Autodesk Inventor part; units mm, degrees
ref_plane "YZ Plane" through (0, 0, 0) normal (1, 0, 0) x (0, 1, 0)
ref_plane "XZ Plane" through (0, 0, 0) normal (0, 1, 0) x (-1, 0, 0)
ref_plane "XY Plane" through (0, 0, 0) normal (0, 0, 1) x (1, 0, 0)
sketch "Sketch1" plane through (0, 0, 0) normal (0, 1, 0) x (-1, 0, 0)
  circle A0 centre (0, 0) radius 1.651
  circle A1 centre (0, -101.1428) radius 1.651
  line L0 (0, 0) -> (0, -101.1428) construction
  line L1 (3.175, 3.175) -> (-6.35, 3.175)
  line L2 (-6.35, 3.175) -> (-6.35, -104.3178)
  line L3 (-6.35, -104.3178) -> (3.175, -104.3178)
  line L4 (3.175, -104.3178) -> (3.175, 3.175)
  dimension "d0" = 3.302
  dimension "d1" = 101.1428
  dimension "d3" = 3.175
  dimension "d4" = 3.175
  dimension "d5" = 3.175
  dimension "d6" = 6.35
extrude "Extrusion1" add sketch "Sketch1" along normal blind 3.175
sketch "Sketch2" plane through (0, 0, 0) normal (0, -1, 0) x (1, 0, 0)
  line L0 (6.35, 3.175) -> (6.35, -104.3178)
  line L1 (6.35, -31.5214) -> (3.175, -31.5214)
  line L2 (3.175, -31.5214) -> (3.175, -69.6214)
  line L3 (3.175, -69.6214) -> (6.35, -69.6214)
  line L4 (6.35, -69.6214) -> (6.35, -31.5214)
  line L5 (-3.175, -104.3178) -> (-3.175, 3.175) construction
  line L6 (-3.175, -50.5714) -> (6.35, -50.5714) construction
  point P0 (0, 0)
  dimension "d9" = 38.1
  dimension "d10" = 3.175
extrude "Extrusion2" add sketch "Sketch2" along normal blind 41.275
sketch "Sketch3" plane through (6.35, 0, -104.3178) normal (1, 0, 0) x (0, 0, -1)
  circle A0 centre (-70.5866, -39.0652) radius 1.27
  circle A1 centre (-70.5866, -11.5697) radius 1.27
  circle A2 centre (-36.9062, -11.5697) radius 1.27
  circle A3 centre (-36.9062, -39.0652) radius 1.27
  line L0 (-70.5866, -11.5697) -> (-70.5866, -39.0652) construction
  line L1 (-70.5866, -39.0652) -> (-36.9062, -39.0652) construction
  line L2 (-36.9062, -39.0652) -> (-36.9062, -11.5697) construction
  line L3 (-36.9062, -11.5697) -> (-70.5866, -11.5697) construction
  line L4 (-34.6964, -41.275) -> (-72.7964, -41.275) construction
  line L5 (-53.7464, -41.275) -> (-53.7464, 0) construction
  line L6 (-34.6964, 0) -> (-72.7964, 0) construction
  line L7 (-68.3768, -41.275) -> (-39.116, -41.275)
  line L8 (-39.116, -41.275) -> (-39.116, -3.175)
  line L9 (-39.116, -3.175) -> (-68.3768, -3.175)
  line L10 (-68.3768, -3.175) -> (-68.3768, -41.275)
  line L11 (-72.7964, 0) -> (-72.7964, -41.275)
  point P0 (-104.3178, 0)
  dimension "d13" = 2.54
  dimension "d14" = 27.4955
  dimension "d15" = 33.6804
  dimension "d17" = 2.2098
  dimension "d18" = 2.2098
  dimension "d19" = 2.2098
  dimension "d20" = 2.2098
  dimension "d21" = 3.175
extrude "Extrusion3" cut sketch "Sketch3" against normal up to surface (3.175 mm away)
chamfer "Chamfer1" distance 6.35 angle 45 1 edges at (3.175, 0, -50.5714)
chamfer "Chamfer2" distance 3.175 distance2 34.6964 1 edges at (6.35, 1.5875, 3.175) measured on face at (0, 1.0583, 3.175)
chamfer "Chamfer3" distance 34.6964 distance2 3.175 1 edges at (6.35, 1.5875, -104.3178) measured on face at (6.35, 2.1167, -68.4869)
properties part number "grumpy camera mount"
Can you work these out from the model? Positions are in its coordinate system, mm. A direction names the side the tool comes from. Give positions to 0.01 mm unless a question says otherwise; leave off trailing zeros. Write each loop counter-clockwise with the first axis right and the second up, starting at its lowest first coordinate (ties: lowest second). Pieces come first, ordered by that corner, then holes. Notation, with made-up numbers: M 40,79.5 L 59,79.5 A6 ccw 59,88.5 Z; hole C 30.25,14.5 d9. An arc over 180 degrees is marked long. Answer in a Markdown table with one row per item. Add a question column.
Item 1: On a 3-axis mill with a long thin cutter (end or side, diameter ignored), from which of +Z, -Z, +X, -X, +Y, -Y can I reach the whole of each face in a straight line? I mean faces 4 (the flat face through (3, -3.175, -51)), 5 (the flat face through (3.175, -24, -34)), 6 (the flat face through (5, -16, -69.621)). Say none if no direction works.
Item 2: Imagine slicing it at B-B, the plane z = 0. Write out the boundary of the cut face in (x, y) (3 decimals).
Item 3: Imagine slicing it at D-D, the plane z = -39.5. Write out the boundary of the cut face in (x, y) (3 decimals), plus the area to 3 significant figures.
Item 4: We'd pull the mould along X, two halves only. Please class faces 1 (the cylindrical face through (-1.525, 1.565, 0.632)), 2 (the flat face through (3.175, -24, -67)), 3 (the flat face through (5, -22, -65.202)): released by +X, released by -X, zero draft, split by the parting line, or undercut.
Item 5: Imagine slicing it at A-A, the plane y = -20. Write out the boundary of the cut face in (x, z) (3 decimals), plus the area to 3 significant figures.
Item 6: For pin 1 Ø3 at (x, z) = (0.5, -19) entering from -Y; pin 2 Ø8 at (y, z) = (-22.5, -62.5) entering from -X (3 decimals); pin 3 Ø1.9 at (x, y) = (2.5, -29.5) entering from +Z, each with a flat end and sliding along its axis, tell me the tip position at first contact or that it passes through.
Item 7: Please list where these lines run through material, in increasing order: L1, parallel to Z at x = 0, y = 1.5 (3 decimals); L2, parallel to Z at x = 6, y = -18; L3, parallel to Y at x = 5, z = -68.5 (3 decimals).
Item 8: Imagine slicing it at C-C, the plane x = 5.25. Write out the boundary of the cut face in (y, z) (3 decimals).
Evaluation:
| question | item | result |
|---|---|---|
| 1 | face 4 | +X, -X, -Y |
| 1 | face 5 | +Z, -Z, -X, -Y |
| 1 | face 6 | -Z, +X, -X, -Y |
| 2 | outline | M -3.175,0 L -1.651,0 L -1.651,3.175 L -3.175,3.175 Z; M 1.651,0 L 3.466,0 L 3.466,3.175 L 1.651,3.175 Z |
| 3 | outline | M -3.175,0 L 0,-3.175 L 6.35,-3.175 L 6.35,3.175 L -3.175,3.175 Z |
| 3 | area | 55.4 mm² |
| 4 | face 1 | undercut |
| 4 | face 2 | released by -X |
| 4 | face 3 | zero draft |
| 5 | outline | M 3.175,-69.621 L 6.35,-69.621 L 6.35,-65.202 L 3.175,-65.202 Z; M 3.175,-35.941 L 6.35,-35.941 L 6.35,-31.521 L 3.175,-31.521 Z |
| 5 | area | 28.1 mm² |
| 6 | pin 1 | stops at y = 0 |
| 6 | pin 2 | stops at x = 3.175 |
| 6 | pin 3 | stops at z = -31.52 |
| 7 | L1 | z = -104.318 to -102.794, -99.492 to -1.651, 1.651 to 3.175 |
| 7 | L2 | z = -69.62 to -65.2, -35.94 to -31.52 |
| 7 | L3 | y = -41.275 to -39.72, -38.411 to -12.224, -10.915 to 3.175 |
| 8 | outline | M -41.275,-69.621 L 0,-69.621 L 0,-81.642 L 3.175,-81.642 L 3.175,-19.501 L 0,-19.501 L 0,-31.521 L -41.275,-31.521 L -41.275,-35.941 L -3.175,-35.941 L -3.175,-65.202 L -41.275,-65.202 Z; hole C -39.065,-67.412 d2.54; hole C -39.065,-33.731 d2.54; hole C -11.57,-67.412 d2.54; hole C -11.57,-33.731 d2.54 |
